Check sheet for the modelled part. Datum: model origin and axes. Units: mm. A direction names the side the tool comes from. Coordinates: 2 decimals unless noted, no trailing zeros. Write each loop counter-clockwise with the first axis right and the second up, starting at its lowest first coordinate (ties: lowest second). Pieces come first, ordered by that corner, then holes. Notation, with made-up numbers: (70.25, 50.25) -> (104.25, 50.25) arc R27 cw to (104.25, 81.25) -> close; hole circle Ø5 at (56, 51.5). An arc over 180 degrees is marked (long way). One line per item, written item: value. Start each with the question number.
1) Scan lines: line 1 along Y through (x, z) = (-68.58, 0.75); line 2 along Y through (x, z) = (-36.83, 7.75); line 3 along Y through (x, z) = (-28, 7.25). Record each from-to range of solid material in increasing order. Write a range as [from, to].
2) Sectioned sample at D-D on y = 12. Enter the section's corners in (x, z).
3) Draft check along Y on faces 1 (the flat face through (-16.51, 44, 7)), 2 (the flat face through (-49, 0, 1)), 3 (the flat face through (-15, 40.005, 7)). Enter one of: +Y half, -Y half, draft (parallel to the pull), parting line (faces both ways), or undercut.
4) Sectioned sample at A-A on z = 3. Give the number of separate pieces and of enclosed holes in the cut face, plus the area to 3 significant figures.
5) Set-up check for faces 4 (the flat face through (-13.97, 31, 7)), 5 (the flat face through (-38, 33.02, 4)), 6 (the flat face through (-38, 17, 5.626)), 7 (the flat face through (-15, 34.925, 7)), 8 (the flat face through (-40.42, 58, 6)): record each of +Z, -Z, +X, -X, +Y, -Y from which the full face is reachable in a straight line by a thin tool's end or side.
6) Gauge pin test, flat ends, axial feed: P1, Ø10, axis at x = -24.5, y = 15, coming from the +Z side; P2, Ø5, axis at x = -68.5, z = 6.5, coming from the -Y side; P3, Ø1.5, axis at x = -56.5, y = 20, coming from the +Z side; P4, Ø2, axis at x = -15.5, z = 6, coming from the -Y side (3 decimals). Record the tip position at first contact, or that the pin passes through.
7) Sectioned sample at B-B on x = -92.71. Enter the section's corners in (y, z).
```python
from build123d import *

# Parameters (mm, degrees)
SKETCH1_W            = 96.52
SKETCH1_H            = 63.5
BOSS_EXTRUDE1_DEPTH  = 1.5875
SKETCH2_R            = 0.5842
SKETCH2_R_2          = 1.524
SKETCH2_R_3          = 0.508
HOLES_DEPTH          = 116.54601056
SKETCH3_W            = 17.78
SKETCH3_H            = 33.02
PRO_MICRO_DEPTH      = 4.0386
SKETCH4_R            = 1.524
MOUNTING_HOLES_DEPTH = 116.605668935
SKETCH5_W            = 12.5
SKETCH5_H            = 7.62
SKETCH5_R            = 0.5
DC_RELAY_DEPTH       = 9.85
SKETCH6_W            = 2.54
SKETCH6_H            = 7.62
BOSS_EXTRUDE2_DEPTH  = 11.1125


with BuildPart() as part:
    # Sketch1 → Boss-Extrude1 (new body)
    with BuildSketch(Plane.XY):
        with Locations((-48.26, 31.75)):
            Rectangle(SKETCH1_W, SKETCH1_H)
    extrude(amount=BOSS_EXTRUDE1_DEPTH)

    # Sketch2 → Holes (cut, through all)
    with BuildSketch(Plane.XY.offset(1.5875)):
        with Locations((-68.58, 5.08)):
            Circle(SKETCH2_R)
        with Locations((-50.8, 34.29)):
            Circle(SKETCH2_R_2)
        with Locations((-15.24, 46.355)):
            Circle(SKETCH2_R_3)
        with Locations((-15.24, 43.815)):
            Circle(SKETCH2_R_3)
        with Locations((-15.24, 41.275)):
            Circle(SKETCH2_R_3)
        with Locations((-15.24, 33.655)):
            Circle(SKETCH2_R_3)
        with Locations((-15.24, 31.115)):
            Circle(SKETCH2_R_3)
        with Locations((-15.24, 28.575)):
            Circle(SKETCH2_R_3)
    extrude(amount=-HOLES_DEPTH, mode=Mode.SUBTRACT)

    # Sketch3 → pro micro (add)
    with BuildSketch(Plane.XY.offset(1.5875)):
        with Locations((-38.0492, 16.51)):
            Rectangle(SKETCH3_W, SKETCH3_H)
    extrude(amount=PRO_MICRO_DEPTH)

    # Sketch4 → mounting holes (cut, through all)
    with BuildSketch(Plane.XY.offset(1.5875)):
        with Locations((-92.71, 3.81)):
            Circle(SKETCH4_R)
        with Locations((-92.71, 59.69)):
            Circle(SKETCH4_R)
        with Locations((-3.81, 59.69)):
            Circle(SKETCH4_R)
        with Locations((-3.81, 3.81)):
            Circle(SKETCH4_R)
    extrude(amount=-MOUNTING_HOLES_DEPTH, mode=Mode.SUBTRACT)

    # Sketch5 → DC relay (add)
    with BuildSketch(Plane.XY.offset(1.5875)):
        with Locations((-34.17, 58.36)):
            Rectangle(SKETCH5_W, SKETCH5_H)
        with Locations((-39.37, 60.96)):
            Circle(SKETCH5_R, mode=Mode.SUBTRACT)
        with Locations((-39.37, 55.88)):
            Circle(SKETCH5_R, mode=Mode.SUBTRACT)
        with Locations((-36.83, 60.96)):
            Circle(SKETCH5_R, mode=Mode.SUBTRACT)
        with Locations((-29.21, 60.96)):
            Circle(SKETCH5_R, mode=Mode.SUBTRACT)
        with Locations((-36.83, 55.88)):
            Circle(SKETCH5_R, mode=Mode.SUBTRACT)
        with Locations((-29.21, 55.88)):
            Circle(SKETCH5_R, mode=Mode.SUBTRACT)
    extrude(amount=DC_RELAY_DEPTH)

    # Sketch6 → Boss-Extrude2 (add)
    with BuildSketch(Plane.XY.offset(1.5875)):
        with Locations((-15.24, 43.815)):
            Rectangle(SKETCH6_W, SKETCH6_H)
        with Locations((-15.24, 31.115)):
            Rectangle(SKETCH6_W, SKETCH6_H)
    extrude(amount=BOSS_EXTRUDE2_DEPTH)


solid = part.part
```
Answers:
1. line 1: y = [0, 4.5], [5.66, 63.5]
1. line 2: y = [54.55, 55.38], [56.38, 60.46], [61.46, 62.17]
1. line 3: y = [54.55, 62.17]
2. outline: (-96.52, 0) -> (0, 0) -> (0, 1.59) -> (-29.16, 1.59) -> (-29.16, 5.63) -> (-46.94, 5.63) -> (-46.94, 1.59) -> (-96.52, 1.59) -> close
3. face 1: draft
3. face 2: -Y half
3. face 3: undercut
4. separate pieces: 4
4. enclosed holes: 6
4. area: 716 mm2
5. face 4: +Z, +X, +Y, -Y
5. face 5: +Z, -X
5. face 6: +Z, -X, -Y
5. face 7: +Z, +X, -X
5. face 8: +Z, -X, +Y
6. P1: stops at z = 5.63
6. P2: passes through
6. P3: stops at z = 1.59
6. P4: stops at y = 27.305
7. outline: (0, 0) -> (2.29, 0) -> (2.29, 1.59) -> (0, 1.59) -> close; (5.33, 0) -> (58.17, 0) -> (58.17, 1.59) -> (5.33, 1.59) -> close; (61.21, 0) -> (63.5, 0) -> (63.5, 1.59) -> (61.21, 1.59) -> close
